Geometry: final body of the model. Coordinates: model frame, mm. Face numbers are marked on the shaded views. A direction names the side the tool comes from. Round coordinates to 2 decimals unless told otherwise and drop trailing zeros. Write each loop counter-clockwise with the first axis right and the second up, starting at its lowest first coordinate (ties: lowest second). Pieces come first, ordered by that corner, then holes. Notation, with made-up numbers: (11, 54) - (56, 54) arc R23 ccw to (56, 74) - close; hole circle Ø6 at (38.25, 70.5). An arc over 180 degrees is marked (long way). Use a Markdown table: item, result. Add a question column.
```python
from build123d import *

# Parameters (mm, degrees)
SKETCH2_W            = 100
SKETCH2_H            = 100
BOSS_EXTRUDE1_DEPTH  = 12
SKETCH3_R            = 16
CUT_EXTRUDE1_DEPTH   = 10
M6_CLEARANCE_HOLE1_D = 6.4
BOSS_EXTRUDE2_START  = 30
SKETCH17_R           = 5.2
SKETCH17_R_2         = 3.2
BOSS_EXTRUDE2_DEPTH  = 30
CIRPATTERN1_COUNT    = 4
SKETCH18_R           = 14
CUT_EXTRUDE3_DEPTH   = 77.811457479
FILLET1_R            = 2
FILLET2_R            = 7


with BuildPart() as part:
    # Sketch2 → Boss-Extrude1 (new body)
    with BuildSketch(Plane.XY):
        Rectangle(SKETCH2_W, SKETCH2_H)
    extrude(amount=BOSS_EXTRUDE1_DEPTH)

    # Sketch3 → Cut-Extrude1 (cut)
    with BuildSketch(Plane(origin=(0, 0, 0), x_dir=(-1, 0, 0), z_dir=(0, 0, -1))):
        Circle(SKETCH3_R)
    extrude(amount=-CUT_EXTRUDE1_DEPTH, mode=Mode.SUBTRACT)

    # M6 Clearance Hole1 (through all)
    with Locations(Plane(origin=(0, 0, 12), x_dir=(-1, 0, 0), z_dir=(0, 0, 1))):
        with Locations((42.5, -42.5), (-42.5, 42.5), (-42.5, -42.5), (42.5, 42.5)):
            Hole(M6_CLEARANCE_HOLE1_D / 2)

    # Sketch17 → Boss-Extrude2 (add)
    with BuildSketch(Plane(origin=(0, 0, 0), x_dir=(-1, 0, 0), z_dir=(0, 0, -1)).offset(BOSS_EXTRUDE2_START)):
        with Locations((-42.5, 42.5)):
            Circle(SKETCH17_R)
        with Locations(Location((-42.5, 42.5, 0), (0, 0, 180))):
            Circle(SKETCH17_R_2, mode=Mode.SUBTRACT)
    boss_extrude2 = extrude(amount=-BOSS_EXTRUDE2_DEPTH)

    # CirPattern1: Boss-Extrude2 ×4 about axis
    cirpattern1_axis = Axis((0, 0, 0), (0, 0, 1))
    for i in range(1, CIRPATTERN1_COUNT):
        add(boss_extrude2.rotate(cirpattern1_axis, i * 360 / CIRPATTERN1_COUNT))

    # Sketch18 → Cut-Extrude3 (cut, through all)
    with BuildSketch(Plane(origin=(0, 0, 0), x_dir=(-1, 0, 0), z_dir=(0, 0, -1))):
        Circle(SKETCH18_R)
    extrude(amount=-CUT_EXTRUDE3_DEPTH, mode=Mode.SUBTRACT)

    # Fillet1
    fillet1_edges = [part.edges().sort_by_distance(p)[0] for p in [
        (47.7, 42.5, 0),
        (-42.5, 47.7, 0),
        (-47.7, -42.5, 0),
        (42.5, -47.7, 0),
    ]]
    fillet(fillet1_edges, radius=FILLET1_R)

    # Fillet2
    fillet2_edges = [part.edges().sort_by_distance(p)[0] for p in [
        (50, -50, 6),
        (-50, -50, 6),
        (-50, 50, 6),
        (50, 50, 6),
    ]]
    fillet(fillet2_edges, radius=FILLET2_R)


solid = part.part
```
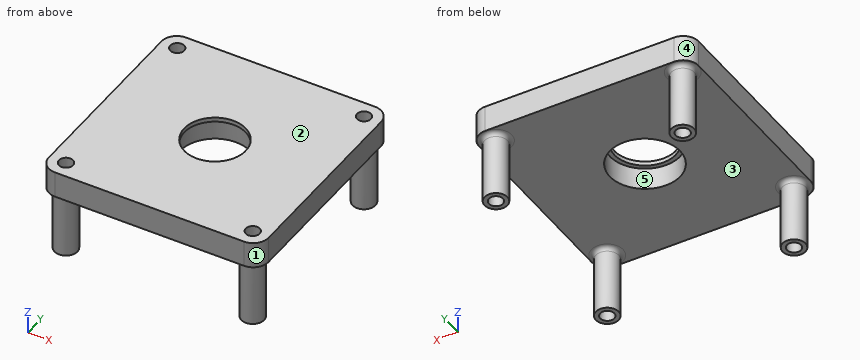
1) Section A-A, the plane z = -17.5. Return the cut outline in (x, y), then the cut area to 3 significant figures.
2) Material intervals for L1, parallel to X at y = 42.5, z = 1; L2, parallel to X at y = -42, z = -10; L3, parallel to Y at x = 0, z = 11.15, sorted ascending. Write a range as from..to.
3) Section B-B, the plane y = 0. Return the cut outline in (x, z), then the cut area to 3 significant figures.
4) Pin query (flat end, axial travel): P1, Ø4, axis at x = 6.5, y = -26.5, coming from the -Z side; P2, Ø17, axis at x = 0, y = 0, coming from the +Z side; P3, Ø2, axis at y = 37, z = -23.5, coming from the -X side. Return the tip coordinate at first contact, or that it passes through.
5) Draft query along X for the marked faces 1, 2 and 3. Return one class per face: released by +X, released by -X, zero draft, split by the parting line, or undercut.
6) Set-up query: the marked faces 4 and 5. Return all of +Z, -Z, +X, -X, +Y, -Y with unobstructed straight access to the full face (end or side cutting, diameter ignored); none if empty.
7) Section C-C, the plane z = 6.5. Return the cut outline in (x, y), then the cut area to 4 significant figures.
Output values:
| question | item | result |
|---|---|---|
| 1 | outline | circle Ø10.4 at (-42.5, -42.5); circle Ø10.4 at (-42.5, 42.5); circle Ø10.4 at (42.5, -42.5); circle Ø10.4 at (42.5, 42.5); hole circle Ø6.4 at (-42.5, -42.5); hole circle Ø6.4 at (-42.5, 42.5); hole circle Ø6.4 at (42.5, -42.5); hole circle Ø6.4 at (42.5, 42.5) |
| 1 | area | 211 mm^2 |
| 2 | L1 | x = -50..-45.7, -39.3..39.3, 45.7..50 |
| 2 | L2 | x = -47.68..-45.66, -39.34..-37.32, 37.32..39.34, 45.66..47.68 |
| 2 | L3 | y = -50..-14, 14..50 |
| 3 | outline | (-50, 0) - (-16, 0) - (-16, 10) - (-14, 10) - (-14, 12) - (-50, 12) - close; (14, 10) - (16, 10) - (16, 0) - (50, 0) - (50, 12) - (14, 12) - close |
| 3 | area | 824 mm^2 |
| 4 | P1 | stops at z = 0 |
| 4 | P2 | passes through |
| 4 | P3 | stops at x = -45.11 |
| 5 | face 1 | released by +X |
| 5 | face 2 | zero draft |
| 5 | face 3 | undercut |
| 6 | face 4 | +Z, -Z, -X, +Y |
| 6 | face 5 | -Z |
| 7 | outline | (-50, -43) arc R7 ccw to (-43, -50) - (43, -50) arc R7 ccw to (50, -43) - (50, 43) arc R7 ccw to (43, 50) - (-43, 50) arc R7 ccw to (-50, 43) - close; hole circle Ø6.4 at (-42.5, -42.5); hole circle Ø6.4 at (-42.5, 42.5); hole circle Ø32 at (0, 0); hole circle Ø6.4 at (42.5, -42.5); hole circle Ø6.4 at (42.5, 42.5) |
| 7 | area | 9,025 mm^2 |
